Could you check a few things on this model? Use its own coordinates, in mm. Face numbers are marked on the shaded views. A direction names the side the tool comes from. Coordinates: 2 decimals unless noted, no trailing zeros. Order: outer loops, then holes, each group sorted by start corner. A loop starts at its lowest first (then second) coordinate and runs counter-clockwise, first axis right, second up. Notation, with made-up numbers: (50.5, -10.5) - (77.5, -10.5) arc R16 cw to (77.5, -2.5) - close; hole circle Ø5 at (13, 10.25). An arc over 180 degrees is marked (long way). One line per item, written item: value.
from build123d import *

# Parameters (mm, degrees)
SKETCH1_W           = 23.6
SKETCH1_H           = 22.88
SKETCH1_R           = 1.525
SKETCH1_W_2         = 3.5
SKETCH1_H_2         = 3.5
BOSS_EXTRUDE1_DEPTH = 3.5
FILLET1_R           = 2


with BuildPart() as part:
    # Sketch1 → Boss-Extrude1 (new body)
    with BuildSketch(Plane.XY):
        with Locations((0, 11.44)):
            Rectangle(SKETCH1_W, SKETCH1_H)
        with Locations((0, 19.38)):
            Circle(SKETCH1_R, mode=Mode.SUBTRACT)
        with Locations((-8.05, 3.75)):
            Rectangle(SKETCH1_W_2, SKETCH1_H_2, mode=Mode.SUBTRACT)
        with Locations((8.05, 3.75)):
            Rectangle(SKETCH1_W_2, SKETCH1_H_2, mode=Mode.SUBTRACT)
        with Locations((8.05, 13.63)):
            Rectangle(SKETCH1_W_2, SKETCH1_H_2, mode=Mode.SUBTRACT)
        with Locations((-8.05, 13.63)):
            Rectangle(SKETCH1_W_2, SKETCH1_H_2, mode=Mode.SUBTRACT)
    extrude(amount=BOSS_EXTRUDE1_DEPTH)

    # Fillet1
    fillet1_edges = [part.edges().sort_by_distance(p)[0] for p in [
        (-11.8, 22.88, 1.75),
        (11.8, 22.88, 1.75),
        (11.8, 0, 1.75),
        (-11.8, 0, 1.75),
    ]]
    fillet(fillet1_edges, radius=FILLET1_R)


solid = part.part
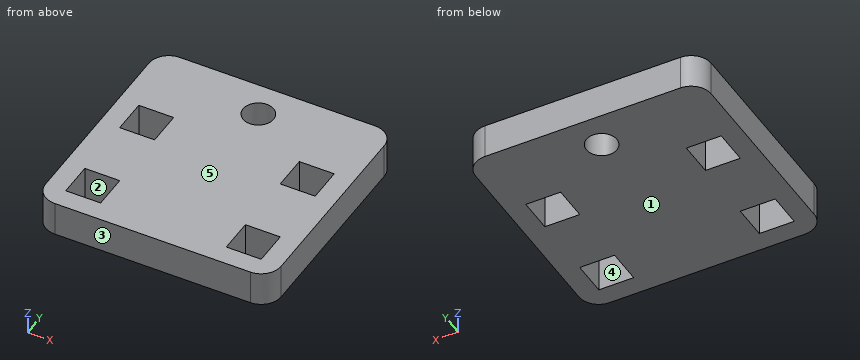
Item 1: Thinking about a two-plate mould opening in Y: for the marked faces 3, 4 and 5, which applies, pulls with the +Y half, pulls with the -Y half, needs draft (parallel to the pull), parting line crosses it, or undercut?
Conclusion:
face 3: pulls with the -Y half
face 4: undercut
face 5: needs draft
Item 2: I want a section at B-B on x = 7.5. Please give me the cut outline in (y, z), then the cut area to 3 significant figures.
Conclusion:
outline: (0, 0) - (2, 0) - (2, 3.5) - (0, 3.5) - close; (5.5, 0) - (11.88, 0) - (11.88, 3.5) - (5.5, 3.5) - close; (15.38, 0) - (22.88, 0) - (22.88, 3.5) - (15.38, 3.5) - close
area: 55.6 mm²
Item 3: I want a section at D-D on x = 0. Please give me the cut outline in (y, z) (3 decimals).
Conclusion:
outline: (0, 0) - (17.855, 0) - (17.855, 3.5) - (0, 3.5) - close; (20.905, 0) - (22.88, 0) - (22.88, 3.5) - (20.905, 3.5) - close
Item 4: I want a section at A-A on y = 14. Please give me the cut outline in (x, z).
Conclusion:
outline: (-11.8, 0) - (-9.8, 0) - (-9.8, 3.5) - (-11.8, 3.5) - close; (-6.3, 0) - (6.3, 0) - (6.3, 3.5) - (-6.3, 3.5) - close; (9.8, 0) - (11.8, 0) - (11.8, 3.5) - (9.8, 3.5) - close
Item 5: For the marked faces 1 and 2, which set-ups out of +Z, -Z, +X, -X, +Y, -Y let a thin tool reach every point of the face, with its end or its side?
Conclusion:
face 1: -Z, +X, -X, +Y, -Y
face 2: +Z, -Z
Item 6: I'm going to push a flat-ended pin straight in: pin 1 Ø12 at (x, y) = (-8, 13.5) entering from +Z. Where does the tip first touch, or does it pass through?
Conclusion:
pin 1: z = 3.5
Item 7: I want a section at C-C on y = 19.38. Please give me the cut outline in (x, z) (3 decimals), then the cut area to 3 significant figures.
Conclusion:
outline: (-11.8, 0) - (-1.525, 0) - (-1.525, 3.5) - (-11.8, 3.5) - close; (1.525, 0) - (11.8, 0) - (11.8, 3.5) - (1.525, 3.5) - close
area: 71.9 mm²
Item 8: If I drill on probe 1 along X at (y, z) = (15.25, 1.4); probe 2 along Y at (x, z) = (-8, 2.15); probe 3 along Y at (x, z) = (0, 1.65) (3 decimals), over which ranges is the centre line in solid material (lowest first)?
Conclusion:
probe 1: -11.8 to -9.8, -6.3 to 6.3, 9.8 to 11.8
probe 2: 0 to 2, 5.5 to 11.88, 15.38 to 22.88
probe 3: 0 to 17.855, 20.905 to 22.88
